Geometry check sheet. Reference: the model listing, model coordinates, mm. Face numbers are marked on the shaded views. A direction names the side the tool comes from. Round coordinates to 2 decimals unless told otherwise and drop trailing zeros. Order: outer loops, then holes, each group sorted by start corner. A loop starts at its lowest first (then second) coordinate and runs counter-clockwise, first axis right, second up.
(1) Release check for a two-part mould opening along Z. For the marked faces 4, 5 and 6 record: +Z half, -Z half, draft (parallel to the pull), parting line (faces both ways), or undercut.
(2) Sectioned sample at C-C (z = -8.5). Give the number of separate pieces and of enclosed holes in the cut face, plus the area to 3 significant figures.
(3) Material ranges on line 1 along Z through (x, y) = (11, -2.25); line 2 along X through (y, z) = (-19.75, -23); line 3 along Z through (x, y) = (27, -12.5), recorded low to high.
(4) Sectioned sample at D-D (z = -21.5). Record the boundary of the cut face in (x, y), plus the area to 3 significant figures.
(5) Set-up check for the marked faces 1, 2 and 3: record each of +Z, -Z, +X, -X, +Y, -Y from which the full face is reachable in a straight line by a thin tool's end or side.
(6) Go/stop test with flat-tipped pins: pin 1 (5 mm diameter, centred on x = 20, z = -10, fed in from +Y); pin 2 (5 mm diameter, centred on x = 15, z = -5.5, fed in from -Y); pin 3 (8 mm diameter, centred on x = 12.5, z = -27, fed in from -Y); pin 4 (0.7 mm diameter, centred on y = -11.5, z = 1.5, fed in from +X). Record where each tip stops, or that it passes through.
(7) Sectioned sample at A-A (y = -21.25). Record the boundary of the cut face in (x, z).
from build123d import *

# Parameters (mm, degrees)
BOSS_EXTRUDE1_DEPTH = 1.778
BOSS_EXTRUDE2_DEPTH = 20.32
SKETCH5_R           = 3.556
SKETCH5_W           = 15.748
SKETCH5_H           = 7.112
CUT_EXTRUDE1_DEPTH  = 1.778
FILLET1_R           = 3.556
SKETCH9_R           = 3.556
BOSS_EXTRUDE3_DEPTH = 2.032
SWEEP2_START        = 13.282231977
SWEEP2_DEPTH        = 14.594268023
CUT_EXTRUDE4_DEPTH  = 0.635
SKETCH17_R          = 2.2225
CUT_EXTRUDE5_DEPTH  = 53.291589362
FILLET2_R           = 0.508
SKETCH19_R          = 2.794
CUT_EXTRUDE6_DEPTH  = 2.54


# Read off the part's stored shape, not the designer's step: Sweep2
with BuildPart() as part:
    # Sketch1 → Boss-Extrude1 (new body)
    with BuildSketch(Plane(origin=(0, 0, 0), x_dir=(1, 0, 0), z_dir=(0, 1, 0))):
        with BuildLine():
            Line((-1.778, 3.3655), (-1.778, 25.8445))
            ThreePointArc((-1.778, 25.8445), (-0.271503729, 29.481503729), (3.3655, 30.988))
            Line((3.3655, 30.988), (27.8765, 30.988))
            ThreePointArc((27.8765, 30.988), (31.513503729, 29.481503729), (33.02, 25.8445))
            Line((33.02, 25.8445), (33.02, 3.3655))
            ThreePointArc((33.02, 3.3655), (31.513503729, -0.271503729), (27.8765, -1.778))
            Line((27.8765, -1.778), (3.3655, -1.778))
            ThreePointArc((3.3655, -1.778), (-0.271503729, -0.271503729), (-1.778, 3.3655))
        make_face()
    extrude(amount=-BOSS_EXTRUDE1_DEPTH)

    # Sketch3 → Boss-Extrude2 (add)
    with BuildSketch(Plane.XZ.offset(1.778)):
        with BuildLine():
            Line((27.8765, 1.778), (3.3655, 1.778))
            ThreePointArc((3.3655, 1.778), (-0.271503729, 0.271503729), (-1.778, -3.3655))
            Line((-1.778, -3.3655), (-1.778, -25.8445))
            ThreePointArc((-1.778, -25.8445), (-0.271503729, -29.481503729), (3.3655, -30.988))
            Line((3.3655, -30.988), (27.8765, -30.988))
            ThreePointArc((27.8765, -30.988), (31.513503729, -29.481503729), (33.02, -25.8445))
            Line((33.02, -25.8445), (33.02, -3.3655))
            ThreePointArc((33.02, -3.3655), (31.513503729, 0.271503729), (27.8765, 1.778))
        make_face()
        with BuildLine():
            Line((0, -3.3655), (0, -25.8445))
            ThreePointArc((0, -25.8445), (0.985732128, -28.224267872), (3.3655, -29.21))
            Line((3.3655, -29.21), (27.8765, -29.21))
            ThreePointArc((27.8765, -29.21), (30.256267872, -28.224267872), (31.242, -25.8445))
            Line((31.242, -25.8445), (31.242, -3.3655))
            ThreePointArc((31.242, -3.3655), (30.256267872, -0.985732128), (27.8765, 0))
            Line((27.8765, 0), (3.3655, 0))
            ThreePointArc((3.3655, 0), (0.985732128, -0.985732128), (0, -3.3655))
        make_face(mode=Mode.SUBTRACT)
    extrude(amount=BOSS_EXTRUDE2_DEPTH)

    # Sketch5 → Cut-Extrude1 (cut)
    with BuildSketch(Plane(origin=(0, 0, 0), x_dir=(1, 0, 0), z_dir=(0, 1, 0))):
        with Locations(Location((24.7269, 5.715, 0), (0, 0, 270))):
            Circle(SKETCH5_R)
        with Locations((11.0109, 5.715)):
            Rectangle(SKETCH5_W, SKETCH5_H)
    extrude(amount=-CUT_EXTRUDE1_DEPTH, mode=Mode.SUBTRACT)

    # Fillet1
    fillet1_edges = [part.edges().sort_by_distance(p)[0] for p in [
        (3.1369, -0.889, -2.159),
        (18.8849, -0.889, -2.159),
        (18.8849, -0.889, -9.271),
        (3.1369, -0.889, -9.271),
    ]]
    fillet(fillet1_edges, radius=FILLET1_R - 0.0001)  # a hair under: the kernel refuses the full size

    # Sketch9 → Boss-Extrude3 (add)
    with BuildSketch(Plane.XZ.offset(1.778)):
        with BuildLine():
            Line((6.6929, -10.541), (15.3289, -10.541))
            ThreePointArc((15.3289, -10.541), (18.327432056, -9.496412634), (20.0279, -6.814852263))
            ThreePointArc((20.0279, -6.814852263), (29.5529, -5.715), (20.0279, -4.615147737))
            ThreePointArc((20.0279, -4.615147737), (18.327432056, -1.933587366), (15.3289, -0.889))
            Line((15.3289, -0.889), (6.6929, -0.889))
            ThreePointArc((6.6929, -0.889), (3.280402674, -2.302502674), (1.8669, -5.715))
            ThreePointArc((1.8669, -5.715), (3.280402674, -9.127497326), (6.6929, -10.541))
        make_face()
        with Locations(Location((24.7269, -5.715, 0), (0, 0, 90))):
            Circle(SKETCH9_R, mode=Mode.SUBTRACT)
        with BuildLine():
            Line((6.6929, -9.271), (15.3289, -9.271))
            ThreePointArc((15.3289, -9.271), (17.843371714, -8.229471714), (18.8849, -5.715))
            ThreePointArc((18.8849, -5.715), (17.843371714, -3.200528286), (15.3289, -2.159))
            Line((15.3289, -2.159), (6.6929, -2.159))
            ThreePointArc((6.6929, -2.159), (4.178428286, -3.200528286), (3.1369, -5.715))
            ThreePointArc((3.1369, -5.715), (4.178428286, -8.229471714), (6.6929, -9.271))
        make_face(mode=Mode.SUBTRACT)
    extrude(amount=BOSS_EXTRUDE3_DEPTH)

    # Sweep1: sweep along a path in Sketch12
    with BuildLine(Plane.XZ.offset(22.098)) as sweep1_path:
        Line((31.242, -25.8445), (31.242, -3.3655))
        ThreePointArc((31.242, -3.3655), (30.256267872, -0.985732128), (27.8765, 0))
        Line((27.8765, 0), (3.3655, 0))
        ThreePointArc((3.3655, 0), (0.985732128, -0.985732128), (0, -3.3655))
        Line((0, -3.3655), (0, -25.8445))
        ThreePointArc((0, -25.8445), (0.985732128, -28.224267872), (3.3655, -29.21))
        Line((3.3655, -29.21), (27.8765, -29.21))
        ThreePointArc((27.8765, -29.21), (30.256267872, -28.224267872), (31.242, -25.8445))
    # Sketch11 → Sweep1 (sweep)
    with BuildSketch(Plane(origin=(0, 0, -9.652), x_dir=(-1, 0, 0), z_dir=(0, 0, -1))):
        Polygon((1.778, -22.098), (0, -22.098), (0.143040428, -23.732959572), align=None)
    sweep(path=sweep1_path.line)

    # Sweep2 outline → Sweep2 (add)
    with BuildSketch(Plane.YZ.offset(SWEEP2_START)):
        Polygon((-17.272, -28.448), (-17.272, -29.21), (-15.494, -29.21), (-16.256, -28.448), align=None)
    extrude(amount=SWEEP2_DEPTH)

    # Sketch16 → Cut-Extrude4 (cut)
    with BuildSketch(Plane.XY.offset(1.778)):
        Polygon((23.045, -16.329), (23.045, -13.369), (21.925, -13.369), (21.925, -8.729), (23.045, -8.729), (23.045, -5.769), (17.493, -5.769), (17.493, -8.729), (18.613, -8.729), (18.613, -11.737), (15.621, -7.642684211), (12.629, -11.737), (12.629, -8.729), (13.749, -8.729), (13.749, -5.769), (8.197, -5.769), (8.197, -8.729), (9.317, -8.729), (9.317, -13.369), (8.197, -13.369), (8.197, -16.329), (12.581, -16.329), (15.621, -12.169), (18.661, -16.329), align=None)
    extrude(amount=-CUT_EXTRUDE4_DEPTH, mode=Mode.SUBTRACT)

    # Sketch17 → Cut-Extrude5 (cut, through all)
    with BuildSketch(Plane(origin=(33.02, 0, 0), x_dir=(0, 0, -1), z_dir=(1, 0, 0))):
        with Locations((13.081, -6.858)):
            Circle(SKETCH17_R)
    extrude(amount=-CUT_EXTRUDE5_DEPTH, mode=Mode.SUBTRACT)

    # Fillet2
    fillet2_edges = [part.edges().sort_by_distance(p)[0] for p in [
        (-1.778, -6.858, -10.8585),
        (31.242, -6.858, -10.8585),
        (0, -6.858, -10.8585),
        (33.02, -6.858, -10.8585),
    ]]
    fillet(fillet2_edges, radius=FILLET2_R)

    # Sketch19 → Cut-Extrude6 (cut)
    with BuildSketch(Plane.ZY.offset(1.778)):
        with Locations((-21.463, -6.4135)):
            Circle(SKETCH19_R)
    extrude(amount=-CUT_EXTRUDE6_DEPTH, mode=Mode.SUBTRACT)

    # Sweep3: sweep along a path in Sketch21
    with BuildLine(Plane(origin=(0, -17.272, 0), x_dir=(-1, 0, 0), z_dir=(0, -1, 0))) as sweep3_path:
        Line((-13.282231977, 0), (-3.3655, 0))
        ThreePointArc((-3.3655, 0), (-0.985732128, 0.985732128), (0, 3.3655))
        Line((0, 3.3655), (0, 16.0655))
    # Sketch20 → Sweep3 (sweep)
    with BuildSketch(Plane(origin=(13.282231977, 0, 0), x_dir=(0, 0, -1), z_dir=(1, 0, 0))):
        Polygon((0, -15.494), (0, -17.272), (0.762, -17.272), (0.762, -16.256), align=None)
    sweep(path=sweep3_path.line)


solid = part.part
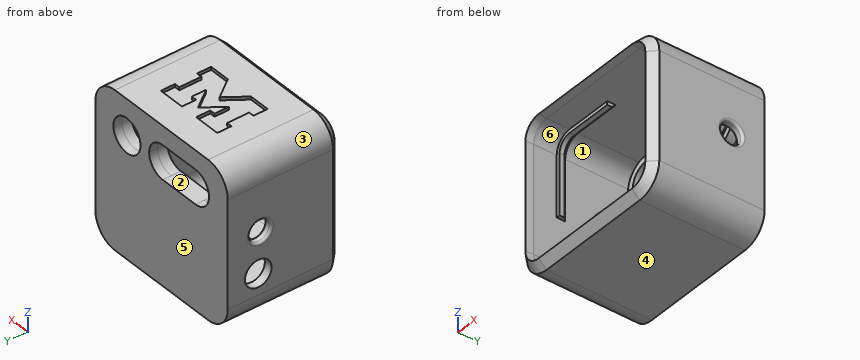
Answer below:
1. face 4: -Z half
1. face 5: draft
1. face 6: undercut
2. separate pieces: 3
2. enclosed holes: 0
2. area: 121 mm2
3. line 1: z = -30.99 to -29.21, -10.54 to -9.27, -2.16 to -0.89, 0 to 1.78
3. line 2: x = -1.78 to 0, 31.24 to 33.02
3. line 3: z = -30.99 to -29.21, 0 to 1.78
4. outline: (-1.78, -22.1) - (-0.14, -23.73) - (0, -22.1) - (0, -9.21) - (-1.78, -9.21) - close; (-1.78, -3.62) - (0, -3.62) - (0, -1.78) - (31.24, -1.78) - (31.24, -22.1) - (31.39, -23.73) - (33.02, -22.1) - (33.02, 0) - (-1.78, 0) - close
4. area: 127 mm2
5. face 1: none
5. face 2: +Y, -Y
5. face 3: +Z, -X, +Y, -Y
6. pin 1: stops at y = 0
6. pin 2: passes through
6. pin 3: stops at y = -23.73
6. pin 4: stops at x = 30.34
7. outline: (-1.78, -25.84) arc R5.14 ccw to (3.37, -30.99) - (27.88, -30.99) arc R5.14 ccw to (33.02, -25.84) - (33.02, -3.37) arc R5.14 ccw to (27.88, 1.78) - (3.37, 1.78) arc R5.14 ccw to (-1.78, -3.37) - close; hole (0, -25.84) arc R3.37 ccw to (3.37, -29.21) - (27.88, -29.21) arc R3.37 ccw to (31.24, -25.84) - (31.24, -3.37) arc R3.37 ccw to (27.88, 0) - (3.37, 0) arc R3.37 ccw to (0, -3.37) - close
